Source: CAD feature listing. Evaluate the final solid. Frame: model axes, mm. A direction names the side the tool comes from. Give positions to 0.01 mm unless a question says otherwise; leave off trailing zeros. Write each loop counter-clockwise with the first axis right and the second up, starting at its lowest first coordinate (ties: lowest second). Pieces come first, ordered by that corner, then holes. Notation, with made-up numbers: (87.5, 52.5) - (140.5, 52.5) arc R15 ccw to (140.5, 80.5) - close; hole circle Ø11 at (-19, -8.75). An arc over 180 degrees is marked (long way). Answer as a JSON object with one key per item and string values. Group by question number.
from build123d import *

# Parameters (mm, degrees)
CYLINDER2357_R              = 1.5
CYLINDER2357_DEPTH          = 20
CYLINDER2367_R              = 1.5
CYLINDER2367_DEPTH          = 20
CYLINDER2363_R              = 1.5
CYLINDER2363_DEPTH          = 20
CYLINDER2378_R              = 1.5
CYLINDER2378_DEPTH          = 20
COMPOUND999_PLACEMENT_ANGLE = 90
CYLINDER2373_R              = 3
CYLINDER2373_DEPTH          = 4
CYLINDER2360_R              = 3
CYLINDER2360_DEPTH          = 4
CYLINDER2362_R              = 3
CYLINDER2362_DEPTH          = 4
CYLINDER2361_R              = 3
CYLINDER2361_DEPTH          = 4
COMPOUND994_PLACEMENT_ANGLE = 90
CYLINDER2359_R              = 10
CYLINDER2359_DEPTH          = 10
CHAMFER057_SIZE             = 2
CUT596_PLACEMENT_ANGLE      = 180


with BuildPart() as obj1:
    # Cylinder2357 → Cylinder2357 (new body)
    with BuildSketch(Plane(origin=(-7, -34, 37), x_dir=(1, 0, 0), z_dir=(0, -1, 0))):
        Circle(CYLINDER2357_R)
    extrude(amount=CYLINDER2357_DEPTH)


with BuildPart() as obj2:
    # Cylinder2367 → Cylinder2367 (new body)
    with BuildSketch(Plane(origin=(7, -34, 73), x_dir=(1, 0, 0), z_dir=(0, -1, 0))):
        Circle(CYLINDER2367_R)
    extrude(amount=CYLINDER2367_DEPTH)


with BuildPart() as obj3:
    # Cylinder2363 → Cylinder2363 (new body)
    with BuildSketch(Plane(origin=(-7, -34, 73), x_dir=(1, 0, 0), z_dir=(0, -1, 0))):
        Circle(CYLINDER2363_R)
    extrude(amount=CYLINDER2363_DEPTH)


with BuildPart() as compound999:
    # Cylinder2378 → Cylinder2378 (new body)
    with BuildSketch(Plane(origin=(7, -34, 37), x_dir=(1, 0, 0), z_dir=(0, -1, 0))):
        Circle(CYLINDER2378_R)
    extrude(amount=CYLINDER2378_DEPTH)

    # Compound999: union obj1, obj2, obj3
    add(obj1.part)
    add(obj2.part)
    add(obj3.part)


with BuildPart() as compound999_1:
    # Compound999 placement: moved
    add(compound999.part.moved(Location((0, 141, 45))).rotate(Axis((0, 141, 45), (1, 0, 0)), COMPOUND999_PLACEMENT_ANGLE))


with BuildPart() as obj4:
    # Cylinder2373 → Cylinder2373 (new body)
    with BuildSketch(Plane(origin=(-7, -34, 37), x_dir=(1, 0, 0), z_dir=(0, -1, 0))):
        Circle(CYLINDER2373_R)
    extrude(amount=CYLINDER2373_DEPTH)


with BuildPart() as obj5:
    # Cylinder2360 → Cylinder2360 (new body)
    with BuildSketch(Plane(origin=(7, -34, 73), x_dir=(1, 0, 0), z_dir=(0, -1, 0))):
        Circle(CYLINDER2360_R)
    extrude(amount=CYLINDER2360_DEPTH)


with BuildPart() as obj6:
    # Cylinder2362 → Cylinder2362 (new body)
    with BuildSketch(Plane(origin=(-7, -34, 73), x_dir=(1, 0, 0), z_dir=(0, -1, 0))):
        Circle(CYLINDER2362_R)
    extrude(amount=CYLINDER2362_DEPTH)


with BuildPart() as compound994:
    # Cylinder2361 → Cylinder2361 (new body)
    with BuildSketch(Plane(origin=(7, -34, 37), x_dir=(1, 0, 0), z_dir=(0, -1, 0))):
        Circle(CYLINDER2361_R)
    extrude(amount=CYLINDER2361_DEPTH)

    # Compound994: union obj4, obj5, obj6
    add(obj4.part)
    add(obj5.part)
    add(obj6.part)


with BuildPart() as compound994_1:
    # Compound994 placement: moved
    add(compound994.part.moved(Location((0, 141, 45))).rotate(Axis((0, 141, 45), (1, 0, 0)), COMPOUND994_PLACEMENT_ANGLE))


with BuildPart() as cut596:
    # Cylinder2359 → Cylinder2359 (new body)
    with BuildSketch(Plane(origin=(0, 106, 0), x_dir=(1, 0, 0), z_dir=(0, 0, 1))):
        Circle(CYLINDER2359_R)
    extrude(amount=CYLINDER2359_DEPTH)

    # Chamfer057
    chamfer057_edges = [cut596.edges().sort_by_distance(p)[0] for p in [
        (-10, 106, 10),
    ]]
    chamfer(chamfer057_edges, length=CHAMFER057_SIZE)

    # Cut595: cut Compound994
    add(compound994_1.part, mode=Mode.SUBTRACT)

    # Cut596: cut Compound999
    add(compound999_1.part, mode=Mode.SUBTRACT)


with BuildPart() as cut596_1:
    # Cut596 placement: moved
    add(cut596.part.moved(Location((52, -19, -36))).rotate(Axis((52, -19, -36), (0, 0, 1)), CUT596_PLACEMENT_ANGLE))


solid = cut596_1.part
Q1. Draft query along Y for faces 3 (the cylindrical face through (59.37, -131.76, -32.06)), 4 (the flat face through (52, -125, -36)), 5 (the flat face through (43.8, -124.3, -29)). Return one class per face: released by +Y, released by -Y, zero draft, split by the parting line, or undercut.
Q2. Reachability of faces 1 (the cylindrical face through (56.148, -123.93, -27.479)), 2 (the cylindrical face through (59.195, -121.513, -32.451)) from +Z, -Z, +X, -X, +Y, -Y: full face, straight path, thin tool, end or side. Return the list, or none.
Q3. Ray query, probe 1 along Z at (x, y) = (60, -125.25); probe 2 along Y at (x, z) = (44.5, -30.25); probe 3 along X at (y, z) = (-123, -32). Return the intervals inside material, ascending. Write a range as [from, to].
Q4. Section A-A on z = -32.25. Return the cut outline in (x, y), then the cut area to 3 significant figures.
Q5. Section B-B on x = 52. Return the cut outline in (y, z).
Q6. First-contact query: pin 1 Ø4 at (y, z) = (-128, -34.5) entering from +X; pin 2 Ø5 at (x, z) = (48.5, -27) entering from +Y; pin 3 Ø2 at (y, z) = (-120, -30.5) entering from -X; pin 4 Ø12 at (x, y) = (59, -119) entering from +Z. Flat tips, straight axial feed; report the tip coordinate or a pass-through.
Q7. Section C-C on y = -125. Return the cut outline in (x, z).
Taken from the geometry:
{
 "1": {"face 3": "split by the parting line", "face 4": "zero draft", "face 5": "undercut"},
 "2": {"face 1": "+Z", "face 2": "+Z, -Z"},
 "3": {"probe 1": "z = [-36, -29]", "probe 2": "y = [-131.61, -124.41], [-121.59, -118.39]", "probe 3": "x = [42.2, 43.5], [46.5, 57.5], [60.5, 61.8]"},
 "4": {"outline": "circle Ø20 at (52, -125); hole circle Ø3 at (45, -123); hole circle Ø3 at (59, -123)", "area": "300 mm²"},
 "5": {"outline": "(-135, -36) - (-115, -36) - (-115, -28) - (-117, -26) - (-133, -26) - (-135, -28) - close"},
 "6": {"pin 1": "stops at x = 61.95", "pin 2": "stops at y = -115.07", "pin 3": "stops at x = 42.83", "pin 4": "stops at z = -26"},
 "7": {"outline": "(42, -36) - (62, -36) - (62, -28) - (61.24, -27.24) - (61.24, -29) - (56.76, -29) - (56.76, -26) - (47.24, -26) - (47.24, -29) - (42.76, -29) - (42.76, -27.24) - (42, -28) - close"}
}
